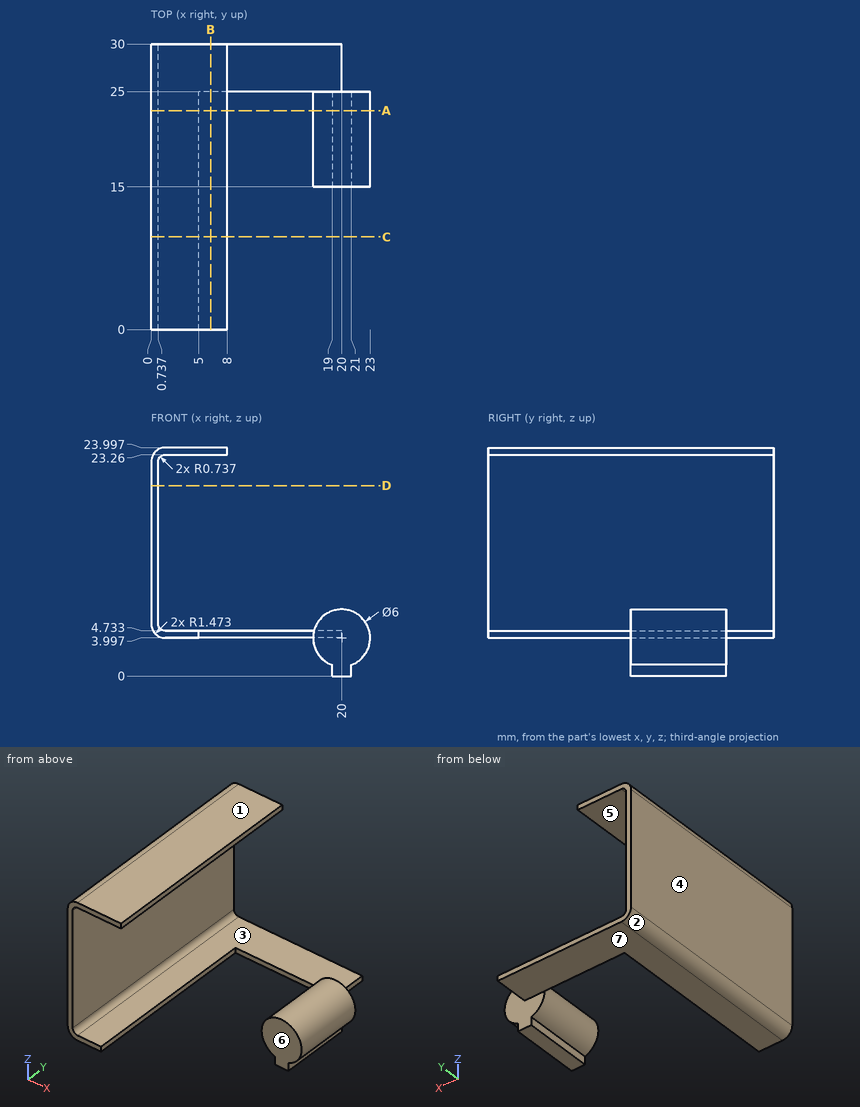
The figure shows three views and two pictorial views of one solid part (mm, origin at its lowest corner). Answer the questions. A direction names the side the tool comes from. Round coordinates to 2 decimals unless told otherwise and drop trailing zeros. Write each loop counter-clockwise with the first axis right and the second up, starting at its lowest first coordinate (ties: lowest second). Pieces come first, ordered by that corner, then holes. Notation, with made-up numbers: (27.25, -6) - (46.25, -6) arc R25 ccw to (46.25, 15) - close; hole circle Ø1 at (15.25, 83.25). An arc over 180 degrees is marked (long way). Answer in a Markdown table with one row per item. Add a question column.
1. A cutting plane is placed at D-D, the plane z = 20. Determine the outline of the cut face in (x, y).
2. Find the intervals of material crossed by line 1 along Z through (x, y) = (3.25, 17.75); line 2 along X through (y, z) = (5, 11); line 3 along Y through (x, z) = (6.25, 4.5), in increasing order. Write a range as from..to.
3. A cutting plane is placed at A-A, the plane y = 23. Determine the outline of the cut face in (x, z).
4. Given pin 1 (1 mm diameter, centred on x = 7.5, y = 4, fed in from -Z); pin 2 (5 mm diameter, centred on x = 19.5, z = 3.5, fed in from -Y); pin 3 (13.5 mm diameter, centred on y = 13.5, z = 17.5, fed in from +X); pin 4 (8 mm diameter, centred on x = 8.5, z = 6.5, fed in from -Y), each flat-ended and moving along its own axis, determine where each tip first touches the part or whether it passes through.
5. The mould has two halves that part along X. Classify the marked faces 1, 2 and 3: +X half, -X half, draft (parallel to the pull), parting line (faces both ways), or undercut.
6. For the marked faces 4, 5, 6 and 7, determine the directions among +Z, -Z, +X, -X, +Y, -Y from which every point of the face is accessible in a straight line to the end or side of a thin tool.
7. A cutting plane is placed at B-B, the plane x = 6.25. Determine the outline of the cut face in (y, z).
8. A cutting plane is placed at C-C, the plane y = 9.75. Determine the outline of the cut face in (x, z).
Worked out:
| question | item | result |
|---|---|---|
| 1 | outline | (0, 0) - (0.74, 0) - (0.74, 30) - (0, 30) - close |
| 2 | line 1 | 4..4.73, 23.26..24 |
| 2 | line 2 | 0..0.74 |
| 2 | line 3 | 25..30 |
| 3 | outline | (0, 5.47) arc R1.47 ccw to (1.47, 4) - (5, 4) - (5, 4.73) - (1.47, 4.73) arc R0.74 cw to (0.74, 5.47) - (0.74, 22.52) arc R0.74 cw to (1.47, 23.26) - (8, 23.26) - (8, 24) - (1.47, 24) arc R1.47 ccw to (0, 22.52) - close; (19, 0) - (21, 0) - (21, 1.17) arc R3 ccw (long way) to (19, 1.17) - close |
| 4 | pin 1 | z = 23.26 |
| 4 | pin 2 | y = 15 |
| 4 | pin 3 | x = 8 |
| 4 | pin 4 | y = 0 |
| 5 | face 1 | draft |
| 5 | face 2 | -X half |
| 5 | face 3 | undercut |
| 6 | face 4 | +Z, -Z, -X, +Y, -Y |
| 6 | face 5 | +X, +Y, -Y |
| 6 | face 6 | +Z, -Z, +X, -Y |
| 6 | face 7 | -Z, -X, +Y |
| 7 | outline | (0, 23.26) - (30, 23.26) - (30, 24) - (0, 24) - close; (25, 4) - (30, 4) - (30, 4.73) - (25, 4.73) - close |
| 8 | outline | (0, 5.47) arc R1.47 ccw to (1.47, 4) - (5, 4) - (5, 4.73) - (1.47, 4.73) arc R0.74 cw to (0.74, 5.47) - (0.74, 22.52) arc R0.74 cw to (1.47, 23.26) - (8, 23.26) - (8, 24) - (1.47, 24) arc R1.47 ccw to (0, 22.52) - close |
